The figure shows three views and two pictorial views of one solid part (mm, origin at its lowest corner). Answer the questions. A direction names the side the tool comes from. Give positions to 0.01 mm unless a question says otherwise; leave off trailing zeros. Write each loop counter-clockwise with the first axis right and the second up, starting at its lowest first coordinate (ties: lowest second). Pieces come first, ordered by that corner, then holes. Notation, with made-up numbers: M -1.75,29.5 L 49.25,29.5 A25 cw 49.25,50.5 Z; hole C 85,74.5 d6. An arc over 180 degrees is marked long. Return JSON: item names as keys, results as strings.
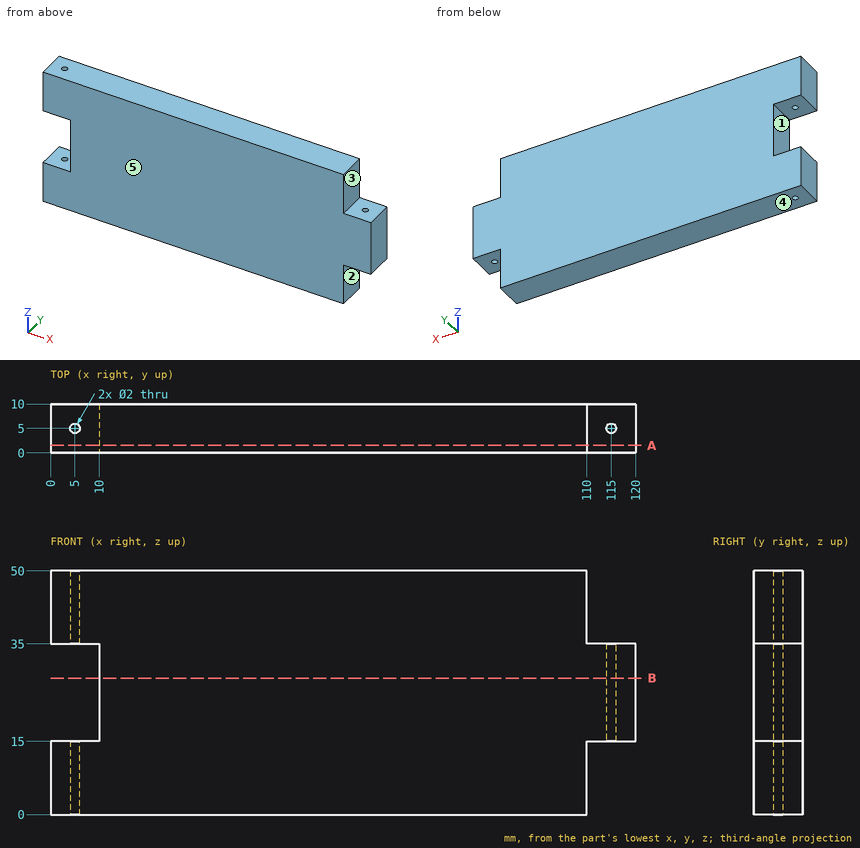
Item 1: Given pin 1 Ø3 at (x, y) = (114.5, 6) entering from -Z; pin 2 Ø5 at (y, z) = (6, 8.5) entering from +X; pin 3 Ø5 at (y, z) = (4.5, 31.5) entering from -X, each flat-ended and moving along its own axis, determine where each tip first touches the part or whether it passes through.
Geometry results:
{"pin 1": "stops at z = 15", "pin 2": "stops at x = 110", "pin 3": "stops at x = 10"}
Item 2: Which of the six approach directions +Z, -Z, +X, -X, +Y, -Y give full straight-line access (tool end or side, diameter ignored) to the marked faces 1, 2, 3, 4 and 5?
Geometry results:
{"face 1": "-X, +Y, -Y", "face 2": "-Z, +X, +Y, -Y", "face 3": "+Z, +X, +Y, -Y", "face 4": "-Z, +X, -X, +Y, -Y", "face 5": "+Z, -Z, +X, -X, -Y"}
Item 3: A cutting plane is placed at A-A, the plane y = 1.5. Write down the section's boundary in (x, z), plus the area to 3 significant figures.
Geometry results:
{"outline": "M 0,0 L 110,0 L 110,15 L 120,15 L 120,35 L 110,35 L 110,50 L 0,50 L 0,35 L 10,35 L 10,15 L 0,15 Z", "area": "5,500 mm2"}
Item 4: Find the intervals of material crossed by line 1 (X direction, y = 5, z = 6.5); line 2 (Y direction, x = 5, z = 6); line 3 (Z direction, x = 8, y = 7.5), in increasing order.
Geometry results:
{"line 1": "x = 0 to 4, 6 to 110", "line 2": "y = 0 to 4, 6 to 10", "line 3": "z = 0 to 15, 35 to 50"}
Item 5: A cutting plane is placed at B-B, the plane z = 28. Write down the section's boundary in (x, y), plus the area to 3 significant figures.
Geometry results:
{"outline": "M 10,0 L 120,0 L 120,10 L 10,10 Z; hole C 115,5 d2", "area": "1,100 mm2"}
